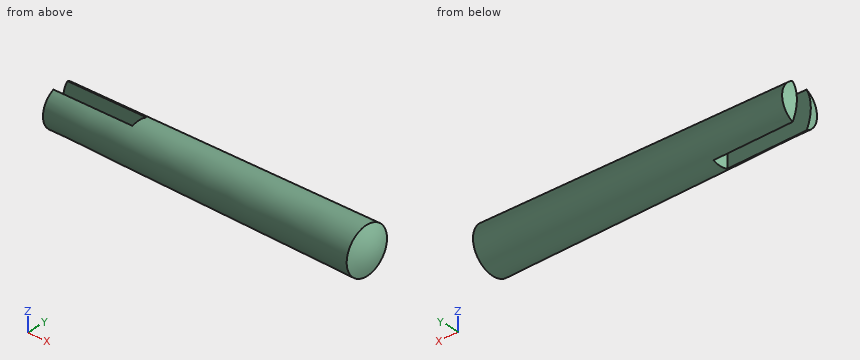
```python
from build123d import *

# Parameters (mm, degrees)
SPLSKE_W      = 5.7748
SPLSKE_H      = 2
SPLIT_2_DEPTH = 30.65250508


with BuildPart() as part:
    # BodySke → Body (revolve)
    with BuildSketch(Plane.XY):
        with BuildLine():
            Line((0.63, 2.5), (39.37, 2.8874))
            ThreePointArc((39.37, 2.8874), (39.840668825, 1.477665283), (40, 0))
            Line((40, 0), (0, 0))
            ThreePointArc((0, 0), (0.159924093, 1.289079129), (0.63, 2.5))
        make_face()
    revolve(axis=Axis((0, 0, 0), (1, 0, 0)))

    # SplSke → Split 2 (cut, through all)
    with BuildSketch(Plane(origin=(10.63, 0, 0), x_dir=(0, 0, -1), z_dir=(1, 0, 0))):
        Rectangle(SPLSKE_W, SPLSKE_H)
    extrude(amount=-SPLIT_2_DEPTH, mode=Mode.SUBTRACT)


solid = part.part
```
Geometry check sheet. Reference: the model listing, model coordinates, mm. Round coordinates to 2 decimals unless told otherwise and drop trailing zeros. Loops run counter-clockwise (first coordinate to the right, second up) from the corner with the lowest first, then second, coordinate; pieces in that order, holes last. Notation, with made-up numbers: M 38,9.5 L 90,9.5 A19 cw 90,44.5 Z; hole C 56.25,50.5 d10. An arc over 180 degrees is marked long. Return JSON: item names as keys, results as strings. Group by question number.
(1) Go/stop test with flat-tipped pins: pin 1 (1.6 mm diameter, centred on y = -0.5, z = -1, fed in from -X); pin 2 (1.5 mm diameter, centred on x = 11.5, y = 0.5, fed in from +Z); pin 3 (2 mm diameter, centred on x = 33, z = 0, fed in from +Y). Record where each tip stops, or that it passes through.
(2) Section check A-A, the plane x = 4. Enter the section's corners in (y, z).
(3) Section check C-C, the plane x = 17.5. Enter the section's corners in (y, z).
(4) Scan lines: line 1 along X through (y, z) = (-0.3, 0.05); line 2 along Y through (x, z) = (3.5, 1.85); line 3 along Y through (x, z) = (5.5, -2.25). Record each from-to range of solid material in increasing order. Write a range as [from, to].
(5) Section check B-B, the plane x = 11. Enter the section's corners in (y, z).
Data:
{
 "1": {"pin 1": "x = 0.11", "pin 2": "z = 2.61", "pin 3": "y = 2.83"},
 "2": {"outline": "M -1,-2.33 L -1,2.33 A2.53 ccw Z; M 1,-2.33 A2.53 ccw 1,2.33 Z"},
 "3": {"outline": "C 0,0 d5.34"},
 "4": {"line 1": "[10.63, 39.99]", "line 2": "[-1.72, -1], [1, 1.72]", "line 3": "[-1.2, -1], [1, 1.2]"},
 "5": {"outline": "C 0,0 d5.21"}
}
